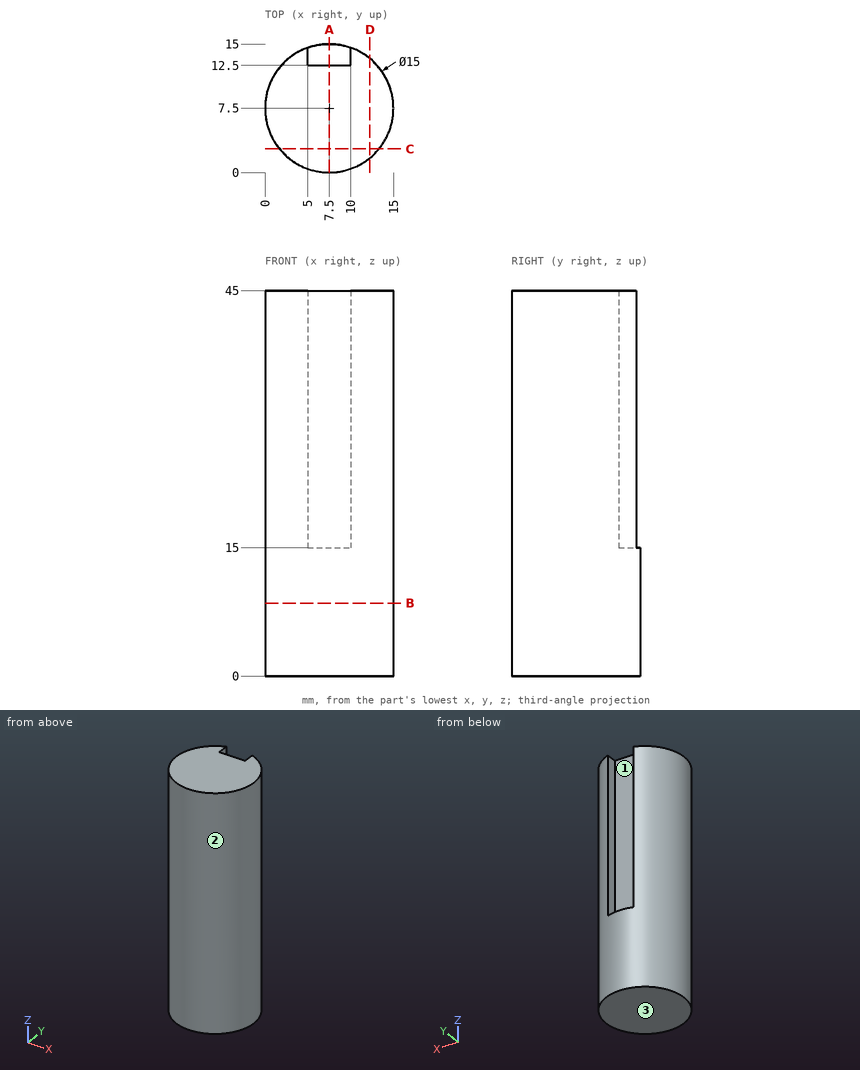
Answer from the drawing. Dimensions are ordinates in mm from the lowest x, y and z of the part. Coordinates: 2 decimals unless noted, no trailing zeros. Loops run counter-clockwise (first coordinate to the right, second up) from the corner with the lowest first, then second, coordinate; pieces in that order, holes last. Notation, with made-up numbers: (4.25, 42.25) - (30.25, 42.25) arc R15 cw to (30.25, 58.25) - close; hole circle Ø5 at (-22, 73.5). An arc over 180 degrees is marked (long way). Answer in a Markdown table with one row per item.
1. Find section B-B, the plane z = 8.5. Write down the section's boundary in (x, y), then the cut area to 3 significant figures.
Conclusion:
| item | result |
|---|---|
| outline | circle Ø15 at (7.5, 7.5) |
| area | 177 mm² |
2. Straight lines are drawn through the part: line 1 (Y direction, x = 7.5, z = 39.5); line 2 (X direction, y = 14, z = 34); line 3 (X direction, y = 13.25, z = 41.5). For each, find the intervals that lie inside material, in ascending order.
Conclusion:
| item | result |
|---|---|
| line 1 | y = 0 to 12.5 |
| line 2 | x = 3.76 to 5, 10 to 11.24 |
| line 3 | x = 2.68 to 5, 10 to 12.32 |
3. Find section A-A, the plane x = 7.5. Write down the section's boundary in (y, z), then the cut area to 3 significant figures.
Conclusion:
| item | result |
|---|---|
| outline | (0, 0) - (15, 0) - (15, 15) - (12.5, 15) - (12.5, 45) - (0, 45) - close |
| area | 600 mm² |
4. Find section C-C, the plane y = 2.75. Write down the section's boundary in (x, z).
Conclusion:
| item | result |
|---|---|
| outline | (1.7, 0) - (13.3, 0) - (13.3, 45) - (1.7, 45) - close |
5. Given pin 1 (2.5 mm diameter, centred on y = 13.5, z = 32.5, fed in from +X); pin 2 (2 mm diameter, centred on x = 8, y = 14.5, fed in from +Z); pin 3 (1.5 mm diameter, centred on x = 1.5, z = 22, fed in from +Y), each flat-ended and moving along its own axis, determine where each tip first touches the part or whether it passes through.
Conclusion:
| item | result |
|---|---|
| pin 1 | stops at x = 13.3 |
| pin 2 | stops at z = 15 |
| pin 3 | stops at y = 12.86 |
6. Determine the mould class of the marked faces 1, 2 and 3 for opening direction X: +X half, -X half, draft (parallel to the pull), parting line (faces both ways), or undercut.
Conclusion:
| item | result |
|---|---|
| face 1 | undercut |
| face 2 | parting line |
| face 3 | draft |
